```python
from build123d import *

# Parameters (mm, degrees)
F0_R     = 1
F1_DEPTH = 3


with BuildPart() as f1:
    # F0 (on Right) → F1 (new body)
    with BuildSketch(Plane.YZ):
        Polygon((-20, 0), (0, 0), (0, 7), (-3, 7), (-3, 17), (0, 17), (0, 24), (-3, 24), (-3, 34), (0, 34), (0, 41), (-20, 41), (-20, 38), (-30, 38), (-30, 41), (-50, 41), (-50, 38), (-55, 38), (-60, 38), (-60, 41), (-80, 41), (-80, 38), (-90, 38), (-90, 41), (-110, 41), (-110, 34), (-107, 34), (-107, 24), (-110, 24), (-110, 17), (-107, 17), (-107, 7), (-110, 7), (-110, 0), (-90, 0), (-90, 3), (-80, 3), (-80, 0), (-60, 0), (-60, 3), (-55, 3), (-50, 3), (-50, 0), (-30, 0), (-30, 3), (-20, 3), align=None)
        with Locations((-70, 1.5)):
            Circle(F0_R, mode=Mode.SUBTRACT)
        with Locations((-40, 1.5)):
            Circle(F0_R, mode=Mode.SUBTRACT)
        with Locations((-70, 39.5)):
            Circle(F0_R, mode=Mode.SUBTRACT)
        with Locations((-40, 39.5)):
            Circle(F0_R, mode=Mode.SUBTRACT)
    extrude(amount=F1_DEPTH)


solid = f1.part
```
Build history of the part. All positions in model axes, mm. A direction names the side the tool comes from. Round coordinates to 2 decimals unless told otherwise and drop trailing zeros. Loops run counter-clockwise (first coordinate to the right, second up) from the corner with the lowest first, then second, coordinate; pieces in that order, holes last.
Item 1: Saw through at C-C (x = 1.95). State how many separate pieces and enclosed holes the cut face has, then the cut area to 3 significant figures.
Item 2: Which spindle directions (+Z, -Z, +X, -X, +Y, -Y) get a long thin tool onto all of the face, cutting with end or side? Do faces 5 (the face through (1, -2, 17)), 6 (the face through (1, -108, 24)), 7 (the face through (1, -80, 40)), 8 (the face through (1, -25, 3)). Say none if no direction does.
Item 3: Two-plate mould, pull along Z, no slides. Class faces 1 (the face through (1, -110, 21)), 2 (the face through (1.479, -39.046, 1.8)), 3 (the face through (1, -2, 34)), 4 (the face through (1, -100, 0)): released by +Z, released by -Z, zero draft, split by the parting line, or undercut.
Item 4: Saw through at D-D (y = -28.5). List the corners of the cut face in (x, z).
Item 5: Saw through at A-A (y = -70). List the corners of the cut face in (x, z).
Item 6: Pin check, flat tips, straight feed: P1, Ø0.9, axis at x = 1.5, y = -86, coming from the +Z side; P2, Ø1, axis at x = 1.5, z = 29.5, coming from the -Y side. Stop position of each tip, or through.
Item 7: Drill centre lines: line 1 along Z through (x, y) = (1.05, -70); line 2 along Z through (x, y) = (0.25, -69.5); line 3 along Y through (x, z) = (1.9, 39). Where is each one in solid material? Low to high.
Item 8: Saw through at B-B (z = 39.5). List the corners of the cut face in (x, y).
Worked answers:
1. separate pieces: 1
1. enclosed holes: 4
1. area: 4,200 mm2
2. face 5: +X, -X, +Y
2. face 6: +X, -X, -Y
2. face 7: +Z, +X, -X
2. face 8: -Z, +X, -X
3. face 1: zero draft
3. face 2: undercut
3. face 3: undercut
3. face 4: released by -Z
4. outline: (0, 3) - (3, 3) - (3, 38) - (0, 38) - close
5. outline: (0, 0) - (3, 0) - (3, 0.5) - (0, 0.5) - close; (0, 2.5) - (3, 2.5) - (3, 38.5) - (0, 38.5) - close; (0, 40.5) - (3, 40.5) - (3, 41) - (0, 41) - close
6. P1: stops at z = 38
6. P2: stops at y = -107
7. line 1: z = 0 to 0.5, 2.5 to 38.5, 40.5 to 41
7. line 2: z = 0 to 0.63, 2.37 to 38.63, 40.37 to 41
7. line 3: y = -110 to -90, -80 to -70.87, -69.13 to -60, -50 to -40.87, -39.13 to -30, -20 to 0
8. outline: (0, -110) - (3, -110) - (3, -90) - (0, -90) - close; (0, -80) - (3, -80) - (3, -71) - (0, -71) - close; (0, -69) - (3, -69) - (3, -60) - (0, -60) - close; (0, -50) - (3, -50) - (3, -41) - (0, -41) - close; (0, -39) - (3, -39) - (3, -30) - (0, -30) - close; (0, -20) - (3, -20) - (3, 0) - (0, 0) - close
